Here's how the part is built. I have some questions about the finished solid (model axes, mm). Give positions to 0.01 mm unless a question says otherwise; leave off trailing zeros. Write each loop counter-clockwise with the first axis right and the second up, starting at its lowest first coordinate (ties: lowest second). Pieces come first, ordered by that corner, then holes. Notation, with made-up numbers: (41.5, 73) - (67.5, 73) arc R24 cw to (67.5, 85) - close; hole circle Ø11 at (3, -7.75). An arc over 180 degrees is marked (long way). Use a Markdown table: item, result.
```python
from build123d import *

# Parameters (mm, degrees)
BOSS_EXTRUDE1_DEPTH = 2.8


with BuildPart() as part:
    # Sketch1 → Boss-Extrude1 (new body)
    with BuildSketch(Plane.XY):
        with BuildLine():
            Line((22.037686993, 65.84113938), (45.437304164, 55.908591182))
            Line((45.437304164, 55.908591182), (75.406514927, 34.923923891))
            Line((75.406514927, 34.923923891), (55.331959214, 11))
            Line((55.331959214, 11), (4.062529555, 11))
            Line((4.062529555, 11), (3.78501031, 28.61298402))
            Line((3.78501031, 28.61298402), (10.294447393, 30.467578469))
            Line((10.294447393, 30.467578469), (11.506283895, 47.384777536))
            Line((11.506283895, 47.384777536), (9.135004308, 52.267647945))
            ThreePointArc((9.135004308, 52.267647945), (10.882479022, 63.525792844), (22.037686993, 65.84113938))
        make_face()
        with BuildLine():
            Line((43.487383815, 52.390841754), (69.536418824, 34.151111078))
            Line((69.536418824, 34.151111078), (53.466728581, 15))
            Line((53.466728581, 15), (8, 15))
            Line((8, 15), (7.832869461, 25.60707524))
            Line((7.832869461, 25.60707524), (14.08410383, 27.388105521))
            Line((14.08410383, 27.388105521), (15.572640754, 48.168033695))
            Line((15.572640754, 48.168033695), (12.733152868, 54.015025105))
            ThreePointArc((12.733152868, 54.015025105), (13.781637696, 60.769912045), (20.474762479, 62.159119966))
            Line((20.474762479, 62.159119966), (43.487383815, 52.390841754))
        make_face(mode=Mode.SUBTRACT)
    extrude(amount=BOSS_EXTRUDE1_DEPTH)


solid = part.part
```
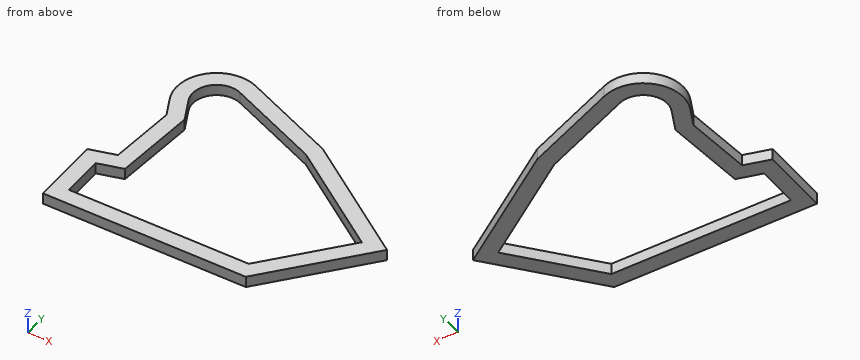
Item 1: If we section it at B-B, the plane y = 61: Write out the boundary of the cut face in (x, z), plus the area to 3 significant figures.
Values:
| item | result |
|---|---|
| outline | (9.13, 0) - (14.01, 0) - (14.01, 2.8) - (9.13, 2.8) - close; (23.21, 0) - (33.44, 0) - (33.44, 2.8) - (23.21, 2.8) - close |
| area | 42.3 mm2 |
Item 2: If we section it at C-C, the plane x = 30: Write out the boundary of the cut face in (y, z).
Values:
| item | result |
|---|---|
| outline | (11, 0) - (15, 0) - (15, 2.8) - (11, 2.8) - close; (58.12, 0) - (62.46, 0) - (62.46, 2.8) - (58.12, 2.8) - close |
Item 3: If we section it at A-A, the plane z = 1.05: Write out the boundary of the cut face in (x, y) (3 decimals).
Values:
| item | result |
|---|---|
| outline | (3.785, 28.613) - (4.063, 11) - (55.332, 11) - (75.407, 34.924) - (45.437, 55.909) - (22.038, 65.841) arc R10 ccw to (9.135, 52.268) - (11.506, 47.385) - (10.294, 30.468) - close; hole (7.833, 25.607) - (8, 15) - (53.467, 15) - (69.536, 34.151) - (43.487, 52.391) - (20.475, 62.159) arc R6 ccw to (12.733, 54.015) - (15.573, 48.168) - (14.084, 27.388) - close |
Item 4: Will this pin go through, and if not, where does the flat tip stop? pin 1 Ø1 at (x, z) = (19.5, 0.5) entering from +Y.
Values:
| item | result |
|---|---|
| pin 1 | stops at y = 66.6 |
Item 5: I need wall thicknesses on line 1 along Y through (x, z) = (18.5, 2.5); line 2 along X through (y, z) = (62, 2.35); line 3 along Y through (x, z) = (56.5, 2.3). Which ranges of each line are inside material? Lowest first, please. Write a range as [from, to].
Values:
| item | result |
|---|---|
| line 1 | y = [11, 15], [62.62, 66.63] |
| line 2 | x = [9.69, 15.44], [20.85, 31.09] |
| line 3 | y = [12.39, 18.61], [43.28, 48.16] |
